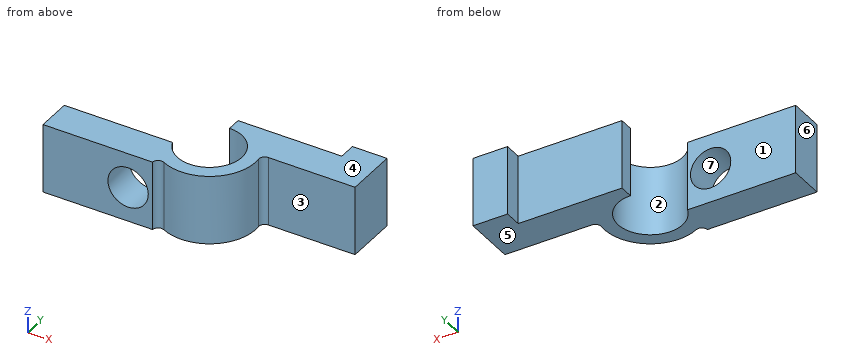
from build123d import *

# Parameters (mm, degrees)
ESBO_O1_R                  = 4
ESBO_O1_W                  = 6.5
ESBO_O1_H                  = 3
EXTRUDE1_CORPO_DEPTH       = 6
FURO_ANEL_DEPTH            = 21.591260282
FURO_ANEL_DEPTH_BACK       = 21.591260282
ESBO_O2_R                  = 2.8
ABERTURA_C_DEPTH           = 21.591260282
ABERTURA_C_DEPTH_BACK      = 21.591260282
ESBO_O3_W                  = 6
ESBO_O3_H                  = 6
FILLET_JUNCOES_R           = 0.5
ESBO_O4_W                  = 6
ESBO_O4_H                  = 3
RESSALTO_EXTRUS_O2_DEPTH   = 3
ESBO_O5_W                  = 6
ESBO_O5_H                  = 3
RESSALTO_EXTRUS_O3_DEPTH   = 3
ESBO_O6_W                  = 3
ESBO_O6_H                  = 6
RESSALTO_EXTRUS_O4_DEPTH   = 1.5
CORTE_EXTRUS_O3_DEPTH      = 23.78705773
CORTE_EXTRUS_O3_DEPTH_BACK = 23.78705773
ESBO_O7_R                  = 1.75


with BuildPart() as part:
    # Esbo_o1 → Extrude1_Corpo (new body)
    with BuildSketch(Plane.XY):
        with BuildLine():
            ThreePointArc((5.127016654, 3), (5.6414319, 1.827439226), (6.5, 0.877501001))
            Line((6.5, 0.877501001), (6.5, 3))
            Line((6.5, 3), (5.127016654, 3))
        make_face()
        with BuildLine():
            ThreePointArc((12.872983346, 5), (11.449489743, 7.16227766), (9, 8))
            Line((9, 8), (9, 5))
            Line((9, 5), (12.872983346, 5))
        make_face()
        with Locations((9, 4)):
            Circle(ESBO_O1_R)
        with Locations((3.25, 1.5)):
            Rectangle(ESBO_O1_W, ESBO_O1_H)
        with BuildLine():
            Line((18, 8), (9, 8))
            ThreePointArc((9, 8), (11.449489743, 7.16227766), (12.872983346, 5))
            Line((12.872983346, 5), (18, 5))
            Line((18, 5), (18, 8))
        make_face()
        with BuildLine():
            Line((6.5, 3), (6.5, 0.877501001))
            ThreePointArc((6.5, 0.877501001), (10.732050808, 0.394448725), (13, 4))
            ThreePointArc((13, 4), (12.968118785, 4.50401717), (12.872983346, 5))
            Line((12.872983346, 5), (9, 5))
            Line((9, 5), (9, 8))
            ThreePointArc((9, 8), (5.83772234, 6.449489743), (5.127016654, 3))
            Line((5.127016654, 3), (6.5, 3))
        make_face()
    extrude(amount=EXTRUDE1_CORPO_DEPTH)

    # Esbo_o2 → Furo_Anel (cut, two sides: drawn at the far end of the back side and taken through both)
    with BuildSketch(Plane(origin=(0, 0, 0), x_dir=(-1, 0, 0), z_dir=(0, 0, -1)).offset(-FURO_ANEL_DEPTH_BACK)):
        with Locations((-9, 4)):
            Circle(ESBO_O2_R)
    extrude(amount=FURO_ANEL_DEPTH + FURO_ANEL_DEPTH_BACK, mode=Mode.SUBTRACT)

    # Esbo_o3 → Abertura_C (cut, two sides: drawn at the far end of the back side and taken through both)
    with BuildSketch(Plane(origin=(0, 0, 0), x_dir=(-1, 0, 0), z_dir=(0, 0, -1)).offset(-ABERTURA_C_DEPTH_BACK)):
        with Locations((-6, 6)):
            Rectangle(ESBO_O3_W, ESBO_O3_H)
    extrude(amount=ABERTURA_C_DEPTH + ABERTURA_C_DEPTH_BACK, mode=Mode.SUBTRACT)

    # Fillet_Juncoes
    # the kernel refuses this fillet: 0.5 mm, written as the material it adds along each edge
    with BuildSketch(Plane(origin=(12.872983346, 5, 0), x_dir=(1, 0, 0), z_dir=(0, 0, 1))) as fillet_juncoes_piece_1:
        with BuildLine():
            CenterArc((0.599152609, -0.5), FILLET_JUNCOES_R, 90, 96.379370208)
            Line((0.102248614, -0.555555556), (0.092310534, -0.556666667))
            ThreePointArc((0.092310534, -0.556666667), (0.051108802, -0.277780632), (-0.009682458, -0.0025))
            Line((-0.009682458, -0.0025), (0, 0.01))
            Line((0, 0.01), (0.599152609, 0.01))
            Line((0.599152609, 0.01), (0.599152609, 0))
        make_face()
    extrude(amount=6)
    with BuildSketch(Plane(origin=(6.5, 0.877501001, 0), x_dir=(0.8430003462487853, -0.5379130191995991, 0), z_dir=(0, 0, 1))) as fillet_juncoes_piece_2:
        with BuildLine():
            CenterArc((0.909219503, -0.497131286), FILLET_JUNCOES_R, 96.140505738, 112.885380476)
            Line((0.472019213, -0.739733648), (0.463275207, -0.744585695))
            ThreePointArc((0.463275207, -0.744585695), (0.227579603, -0.375245954), (-0.008430003, -0.00537913))
            Line((-0.008430003, -0.00537913), (0.00106967, 0.009942626))
            ThreePointArc((0.00106967, 0.009942626), (0.427868002, -0.012949715), (0.854666333, 0.009942626))
            Line((0.854666333, 0.009942626), (0.855736003, 0))
        make_face()
    extrude(amount=6)

    # Esbo_o4 → Ressalto-extrus_o2 (add)
    with BuildSketch(Plane.ZY):
        with Locations((3, 1.5)):
            Rectangle(ESBO_O4_W, ESBO_O4_H)
    extrude(amount=RESSALTO_EXTRUS_O2_DEPTH)



with BuildPart() as body_2:
    # Esbo_o5 → Ressalto-extrus_o3 (new body)
    with BuildSketch(Plane(origin=(18, 0, 0), x_dir=(0, 0, -1), z_dir=(1, 0, 0))):
        with Locations((-3, 6.5)):
            Rectangle(ESBO_O5_W, ESBO_O5_H)
    extrude(amount=RESSALTO_EXTRUS_O3_DEPTH)


with BuildPart() as part_1:
    add(part.part)

    add(body_2.part)  # Ressalto-extrus_o4 merges body 2
    # Esbo_o6 → Ressalto-extrus_o4 (add)
    with BuildSketch(Plane(origin=(0, 8, 0), x_dir=(1, 0, 0), z_dir=(0, 1, 0))):
        with Locations((19.5, -3)):
            Rectangle(ESBO_O6_W, ESBO_O6_H)
    extrude(amount=RESSALTO_EXTRUS_O4_DEPTH)

    # Esbo_o7 → Corte-extrus_o3 (cut, two sides: drawn at the far end of the back side and taken through both)
    with BuildSketch(Plane(origin=(0, 3, 0), x_dir=(1, 0, 0), z_dir=(0, 1, 0)).offset(-CORTE_EXTRUS_O3_DEPTH_BACK)):
        with Locations(Location((4.384660634, -3, 0), (0, 0, 270))):
            Circle(ESBO_O7_R)
    extrude(amount=CORTE_EXTRUS_O3_DEPTH + CORTE_EXTRUS_O3_DEPTH_BACK, mode=Mode.SUBTRACT)


solid = part_1.part
Could you check a few things on this model? Use its own coordinates, in mm. Face numbers are marked on the shaded views. A direction names the side the tool comes from. Give positions to 0.01 mm unless a question says otherwise; leave off trailing zeros. Order: outer loops, then holes, each group sorted by start corner. A loop starts at its lowest first (then second) coordinate and runs counter-clockwise, first axis right, second up.
1. Suppose I cut it at B-B (z = 2.25). List the corners of the cut face in (x, y) for me.
2. For the marked faces 1, 2 and 3, which set-ups out of +Z, -Z, +X, -X, +Y, -Y let a thin tool reach every point of the face, with its end or its side?
3. We'd pull the mould along Z, two halves only. Please class the marked faces 4, 5, 6 and 7: pulls with the +Z half, pulls with the -Z half, needs draft (parallel to the pull), parting line crosses it, or undercut.
4. Suppose I cut it at D-D (z = 0.8). List the corners of the cut face in (x, y) for me.
5. Will these pins go through, and if not, where does the flat tip stop? P1, Ø3, axis at x = 17, z = 2, coming from the -Y side; P2, Ø5, axis at x = 9, y = 4, coming from the +Z side; P3, Ø1.8, axis at x = 4, z = 1.5, coming from the +Y side; P4, Ø3, axis at x = 11.5, z = 1.5, coming from the -Y side.
6. Suppose I cut it at A-A (y = 2.75). List the corners of the cut face in (x, z) for me.
7. I need wall thicknesses on L1, parallel to X at y = 2.5, z = 3.4; L2, parallel to Y at x = 0.5, z = 4.1; L3, parallel to X at y = 7.25, z = 4.75. Which ranges of each line are inside material? Lowest first, please.
8. Suppose I cut it at C-C (x = 10). List the corners of the cut face in (y, z) for me, plus the area to 3 significant figures.
Solved:
1. outline: (-3, 0) - (2.8, 0) - (2.8, 3) - (-3, 3) - close; (5.97, 0) - (6.5, 0) arc R0.5 cw to (7.22, 0.42) arc R4 ccw to (12.98, 4.44) arc R0.5 cw to (13.47, 5) - (21, 5) - (21, 9.5) - (18, 9.5) - (18, 8) - (9, 8) - (9, 6.8) arc R2.8 cw (long way) to (6.38, 3) - (5.97, 3) - close
2. face 1: +Z, -Z, -X, +Y
2. face 2: +Z, -Z
2. face 3: +Z, -Z, +X, -Y
3. face 4: pulls with the +Z half
3. face 5: pulls with the -Z half
3. face 6: needs draft
3. face 7: undercut
4. outline: (-3, 0) - (6.5, 0) arc R0.5 cw to (7.22, 0.42) arc R4 ccw to (12.98, 4.44) arc R0.5 cw to (13.47, 5) - (21, 5) - (21, 9.5) - (18, 9.5) - (18, 8) - (9, 8) - (9, 6.8) arc R2.8 cw (long way) to (6.38, 3) - (-3, 3) - close
5. P1: stops at y = 5
5. P2: passes through
5. P3: stops at y = 3
5. P4: stops at y = 0.13
6. outline: (-3, 0) - (6.49, 0) - (6.49, 6) - (-3, 6) - close; (11.51, 0) - (12.8, 0) - (12.8, 6) - (11.51, 6) - close; hole circle Ø3.5 at (4.38, 3)
7. L1: x = -3 to 2.68, 6.09 to 6.64, 11.36 to 12.71
7. L2: y = 0 to 3
7. L3: x = 9 to 21
8. outline: (0.13, 0) - (1.38, 0) - (1.38, 6) - (0.13, 6) - close; (6.62, 0) - (8, 0) - (8, 6) - (6.62, 6) - close
8. area: 15.9 mm2
